Part model, mm, in its own coordinate system. A direction names the side the tool comes from. Round coordinates to 2 decimals unless told otherwise and drop trailing zeros. Write each loop counter-clockwise with the first axis right and the second up, starting at its lowest first coordinate (ties: lowest second). Pieces come first, ordered by that corner, then holes.
1) Saw through at B-B on z = 38.1. Write the cut outline in (x, y) (3 decimals), and give its area (3 significant figures).
2) Saw through at D-D on y = 16.25. Write the cut outline in (x, z) (3 decimals), and give its area (3 significant figures).
3) Pull direction X, two halves, no side cores. Call faces 3 (the cylindrical face through (12.431, 1.61, 36.048)), 4 (the flat face through (0, 10, 25)), 5 (the flat face through (24, 13, 0)), 6 (the flat face through (3.175, 10, 25)): +X half, -X half, draft (parallel to the pull), parting line (faces both ways), or undercut.
4) Which spindle directions (+Z, -Z, +X, -X, +Y, -Y) get a long thin tool onto all of the face, cutting with end or side? Do faces 1 (the cylindrical face through (1.61, 12.79, 40.17)), 2 (the flat face through (15, 3.175, 25)). Say none if no direction does.
5) Drill centre lines: L1, parallel to X at y = 17.5, z = 38 (3 decimals); L2, parallel to X at y = 23.65, z = 38.1. Where is each one in solid material? Low to high.
6) Saw through at A-A on x = 12.7. Count the separate pieces of the cut face and the enclosed holes in it, and give its area (3 significant figures).
Autodesk Inventor part; units mm, degrees
ref_plane "YZ Plane" through (0, 0, 0) normal (1, 0, 0) x (0, 1, 0)
ref_plane "XZ Plane" through (0, 0, 0) normal (0, 1, 0) x (-1, 0, 0)
ref_plane "XY Plane" through (0, 0, 0) normal (0, 0, 1) x (1, 0, 0)
sketch "Sketch1" plane through (0, 0, 0) normal (0, 0, 1) x (1, 0, 0)
  line L0 (0, 0) -> (25.4, 0)
  line L1 (25.4, 0) -> (25.4, 25.4)
  line L2 (25.4, 25.4) -> (0, 25.4)
  line L3 (0, 25.4) -> (0, 0)
  line L4 (3.175, 22.225) -> (22.225, 22.225)
  line L5 (22.225, 22.225) -> (22.225, 3.175)
  line L6 (22.225, 3.175) -> (3.175, 3.175)
  line L7 (3.175, 3.175) -> (3.175, 22.225)
  dimension "d0" = 25.4
  dimension "d1" = 25.4
  dimension "d2" = 3.175
extrude "Extrusion1" add sketch "Sketch1" along normal blind 50.8
sketch "Sketch2" plane through (25.4, 0, 0) normal (1, 0, 0) x (0, 0, -1)
  line L0 (-50.8, 0) -> (-50.8, 25.4)
  line L1 (0, 0) -> (-50.8, 0)
  circle A0 centre (-38.1, 12.7) radius 2.0701
  circle A1 centre (-25.4, 12.7) radius 2.0701
  circle A2 centre (-12.7, 12.7) radius 2.0701
  dimension "d5" = 4.1402
  dimension "d6" = 12.7
  dimension "d7" = 12.7
  dimension "d10" = 12.7
extrude "Extrusion2" cut sketch "Sketch2" against normal blind 50.8
sketch "Sketch3" plane through (0, 25.4, 0) normal (0, 1, 0) x (1, 0, 0)
  line L0 (25.4, -50.8) -> (0, -50.8)
  line L1 (25.4, 0) -> (25.4, -50.8)
  circle A0 centre (12.7, -38.1) radius 2.0701
  circle A1 centre (12.7, -25.4) radius 2.0701
  circle A2 centre (12.7, -12.7) radius 5.9531
  dimension "d17" = 4.1402
  dimension "d18" = 12.7
  dimension "d19" = 12.7
  dimension "d22" = 12.7
  dimension "d27" = 11.9062
  dimension "d28" = 12.7
  dimension "d29" = 12.7
extrude "Extrusion3" cut sketch "Sketch3" against normal blind 50.8
properties part number "2 in 3-8 in Hex Shaft Holders (4)"
Completed:
1. outline: (0, 0) - (10.63, 0) - (10.63, 3.175) - (3.175, 3.175) - (3.175, 10.63) - (0, 10.63) - close; (0, 14.77) - (3.175, 14.77) - (3.175, 22.225) - (10.63, 22.225) - (10.63, 25.4) - (0, 25.4) - close; (14.77, 0) - (25.4, 0) - (25.4, 10.63) - (22.225, 10.63) - (22.225, 3.175) - (14.77, 3.175) - close; (14.77, 22.225) - (22.225, 22.225) - (22.225, 14.77) - (25.4, 14.77) - (25.4, 25.4) - (14.77, 25.4) - close
1. area: 230 mm2
2. outline: (0, 0) - (3.175, 0) - (3.175, 50.8) - (0, 50.8) - close; (22.225, 0) - (25.4, 0) - (25.4, 50.8) - (22.225, 50.8) - close
2. area: 323 mm2
3. face 3: undercut
3. face 4: -X half
3. face 5: draft
3. face 6: undercut
4. face 1: +X, -X
4. face 2: +Z, -Z
5. L1: x = 0 to 3.175, 22.225 to 25.4
5. L2: x = 0 to 10.63, 14.77 to 25.4
6. separate pieces: 8
6. enclosed holes: 0
6. area: 194 mm2
